```python
from build123d import *

# Parameters (mm, degrees)
SKETCH1_R           = 2.1
SKETCH1_R_2         = 12.5
SKETCH1_R_3         = 2
SKETCH1_R_4         = 2.5
SKETCH1_R_5         = 2.100093489
SKETCH1_R_6         = 2.100208614
SKETCH1_W           = 33
SKETCH1_H           = 80
BOSS_EXTRUDE1_DEPTH = 5


with BuildPart() as part:
    # Sketch1 → Boss-Extrude1 (new body)
    with BuildSketch(Plane.XY):
        with BuildLine():
            Line((101.645117601, -93.770346549), (127.497608455, -93.770346549))
            ThreePointArc((127.497608455, -93.770346549), (132.017726056, -96.632932955), (136.537843658, -93.770346549))
            Line((136.537843658, -93.770346549), (157.551292677, -93.770346549))
            Line((157.551292677, -93.770346549), (157.551292677, 97.083097938))
            Line((157.551292677, 97.083097938), (81.43113923, 97.083097938))
            ThreePointArc((81.43113923, 97.083097938), (77.101012211, 99.583097938), (72.770885192, 97.083097938))
            Line((72.770885192, 97.083097938), (36.650918722, 97.083097938))
            Line((36.650918722, 97.083097938), (-36.650918722, 97.083097938))
            Line((-36.650918722, 97.083097938), (-72.770791704, 97.083097938))
            ThreePointArc((-72.770791704, 97.083097938), (-77.100918722, 99.583097938), (-81.431045741, 97.083097938))
            Line((-81.431045741, 97.083097938), (-157.551292677, 97.083097938))
            Line((-157.551292677, 97.083097938), (-157.551292677, -93.770346549))
            Line((-157.551292677, -93.770346549), (-136.247071986, -93.770346549))
            ThreePointArc((-136.247071986, -93.770346549), (-132.0168916, -96.104718311), (-127.786711214, -93.770346549))
            Line((-127.786711214, -93.770346549), (-101.356014842, -93.770346549))
            ThreePointArc((-101.356014842, -93.770346549), (-97.125834456, -96.104718311), (-92.89565407, -93.770346549))
            Line((-92.89565407, -93.770346549), (-71.59143338, -93.770346549))
            Line((-71.59143338, -93.770346549), (-54.846081626, -64.766546521))
            ThreePointArc((-54.846081626, -64.766546521), (-52.366007385, -62.970931929), (-52.050996654, -59.925317338))
            Line((-52.050996654, -59.925317338), (-36.950417228, -33.770346549))
            Line((-36.950417228, -33.770346549), (36.950417228, -33.770346549))
            Line((36.950417228, -33.770346549), (52.039816857, -59.905953361))
            ThreePointArc((52.039816857, -59.905953361), (52.273889994, -63.173966334), (54.987035679, -65.010686103))
            Line((54.987035679, -65.010686103), (71.59143338, -93.770346549))
            Line((71.59143338, -93.770346549), (92.604882399, -93.770346549))
            ThreePointArc((92.604882399, -93.770346549), (97.125, -96.632932955), (101.645117601, -93.770346549))
        make_face()
        with Locations((20.5, 73.517875823)):
            Circle(SKETCH1_R, mode=Mode.SUBTRACT)
        with Locations((-20.5, 73.517875823)):
            Circle(SKETCH1_R, mode=Mode.SUBTRACT)
        with Locations((0, 73.517875823)):
            Circle(SKETCH1_R_2, mode=Mode.SUBTRACT)
        with Locations((36, 31.229653451)):
            Circle(SKETCH1_R_3, mode=Mode.SUBTRACT)
        with Locations((-5, -3.770346549)):
            Circle(SKETCH1_R_3, mode=Mode.SUBTRACT)
        with Locations((5, -3.770346549)):
            Circle(SKETCH1_R_3, mode=Mode.SUBTRACT)
        with Locations((36, -3.770346549)):
            Circle(SKETCH1_R_3, mode=Mode.SUBTRACT)
        with Locations((-36, 31.229653451)):
            Circle(SKETCH1_R_3, mode=Mode.SUBTRACT)
        with Locations((-5, 31.229653451)):
            Circle(SKETCH1_R_3, mode=Mode.SUBTRACT)
        with Locations((5, 31.229653451)):
            Circle(SKETCH1_R_3, mode=Mode.SUBTRACT)
        with Locations((-36, -3.770346549)):
            Circle(SKETCH1_R_3, mode=Mode.SUBTRACT)
        with Locations((93.2, 39.229653451)):
            Circle(SKETCH1_R_4, mode=Mode.SUBTRACT)
        with Locations((-93.2, 39.229653451)):
            Circle(SKETCH1_R_4, mode=Mode.SUBTRACT)
        with Locations((-93.2, -11.770346549)):
            Circle(SKETCH1_R_4, mode=Mode.SUBTRACT)
        with Locations((93.2, -11.770346549)):
            Circle(SKETCH1_R_4, mode=Mode.SUBTRACT)
        with Locations((-77.100918722, 94.583097938)):
            Circle(SKETCH1_R, mode=Mode.SUBTRACT)
        with Locations((-97.125834456, -91.104718311)):
            Circle(SKETCH1_R, mode=Mode.SUBTRACT)
        with Locations((-55.613602649, -61.095931929)):
            Circle(SKETCH1_R, mode=Mode.SUBTRACT)
        with Locations((77.101012211, 94.583097938)):
            Circle(SKETCH1_R_5, mode=Mode.SUBTRACT)
        with Locations((97.125, -91.632932955)):
            Circle(SKETCH1_R, mode=Mode.SUBTRACT)
        with Locations((55.521485258, -61.298966334)):
            Circle(SKETCH1_R, mode=Mode.SUBTRACT)
        with Locations((-0.000208614, -31.270346549)):
            Circle(SKETCH1_R_6, mode=Mode.SUBTRACT)
        with Locations((-100.592116007, -39.629860895)):
            Circle(SKETCH1_R, mode=Mode.SUBTRACT)
        with Locations((-121.092116007, -75.13690245)):
            Circle(SKETCH1_R, mode=Mode.SUBTRACT)
        with Locations((-110.842116007, -57.383381672)):
            Circle(SKETCH1_R_2, mode=Mode.SUBTRACT)
        with Locations((-132.0168916, -91.104718311)):
            Circle(SKETCH1_R, mode=Mode.SUBTRACT)
        with Locations((132.017726056, -91.632932955)):
            Circle(SKETCH1_R, mode=Mode.SUBTRACT)
        with Locations((121.092116007, -75.13690245)):
            Circle(SKETCH1_R, mode=Mode.SUBTRACT)
        with Locations((100.592116007, -39.629860895)):
            Circle(SKETCH1_R, mode=Mode.SUBTRACT)
        with Locations((110.842116007, -57.383381672)):
            Circle(SKETCH1_R_2, mode=Mode.SUBTRACT)
        with Locations((-56.5, 13.729653451)):
            Rectangle(SKETCH1_W, SKETCH1_H, mode=Mode.SUBTRACT)
        with Locations((56.5, 13.729653451)):
            Rectangle(SKETCH1_W, SKETCH1_H, mode=Mode.SUBTRACT)
        with BuildLine():
            Line((-112.97, 60.222473641), (-115.57, 60.222473641))
            ThreePointArc((-115.57, 60.222473641), (-119.105533906, 58.758007547), (-120.57, 55.222473641))
            Line((-120.57, 55.222473641), (-120.57, -27.763166739))
            ThreePointArc((-120.57, -27.763166739), (-119.105533906, -31.298700645), (-115.57, -32.763166739))
            Line((-115.57, -32.763166739), (-112.97, -32.763166739))
            ThreePointArc((-112.97, -32.763166739), (-109.434466094, -31.298700645), (-107.97, -27.763166739))
            Line((-107.97, -27.763166739), (-107.97, 55.222473641))
            ThreePointArc((-107.97, 55.222473641), (-109.434466094, 58.758007547), (-112.97, 60.222473641))
        make_face(mode=Mode.SUBTRACT)
        with BuildLine():
            Line((112.97, -32.763166739), (115.57, -32.763166739))
            ThreePointArc((115.57, -32.763166739), (119.105533906, -31.298700645), (120.57, -27.763166739))
            Line((120.57, -27.763166739), (120.57, 55.222473641))
            ThreePointArc((120.57, 55.222473641), (119.105533906, 58.758007547), (115.57, 60.222473641))
            Line((115.57, 60.222473641), (112.97, 60.222473641))
            ThreePointArc((112.97, 60.222473641), (109.434466094, 58.758007547), (107.97, 55.222473641))
            Line((107.97, 55.222473641), (107.97, -27.763166739))
            ThreePointArc((107.97, -27.763166739), (109.434466094, -31.298700645), (112.97, -32.763166739))
        make_face(mode=Mode.SUBTRACT)
    extrude(amount=BOSS_EXTRUDE1_DEPTH)


solid = part.part
```
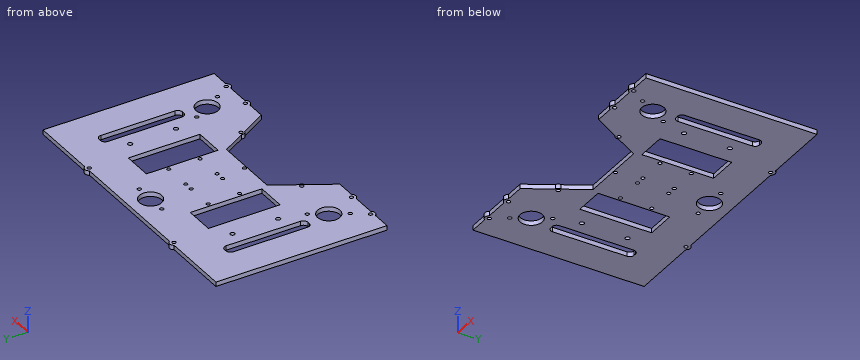
Here's how the part is built. I have some questions about the finished solid (model axes, mm). Give positions to 0.01 mm unless a question says otherwise; leave off trailing zeros. Write each loop counter-clockwise with the first axis right and the second up, starting at its lowest first coordinate (ties: lowest second). Pieces come first, ordered by that corner, then holes. Notation, with made-up numbers: (4, -12) -> (56, -12) arc R24 cw to (56, 12) -> close; hole circle Ø5 at (10, 47.25). An arc over 180 degrees is marked (long way). Write each question's results on one line, items separated by ' | '.
Item 1: Suppose I cut it at B-B on z = 0.9. Give the number of separate pieces and of enclosed holes in the cut face, plus the area to 3 significant figures.
Output:
separate pieces: 1 | enclosed holes: 34 | area: 44,300 mm^2
Item 2: If I drill on L1, parallel to X at y = 34.5, z = 3.7; L2, parallel to Y at x = 36, z = 0.35; L3, parallel to Y at x = -5, z = 2.25, over which ranges is the centre line in solid material (lowest first)?
Output:
L1: x = -157.55 to -120.57, -107.97 to -73, -40 to 40, 73 to 107.97, 120.57 to 157.55 | L2: y = -33.77 to -5.77, -1.77 to 29.23, 33.23 to 97.08 | L3: y = -33.77 to -5.77, -1.77 to 29.23, 33.23 to 62.06, 84.97 to 97.08
Item 3: For pin 1 Ø5 at (x, y) = (-100.59, -39.63) entering from +Z; pin 2 Ø3.5 at (x, y) = (-5, 31.23) entering from -Z; pin 3 Ø1.3 at (x, z) = (114, 2) entering from +Y; pin 4 Ø1.5 at (x, z) = (88.5, 3.5) entering from -Y, each with a flat end and sliding along its axis, tell me the tip position at first contact or that it passes through.
Output:
pin 1: stops at z = 5 | pin 2: passes through | pin 3: stops at y = 97.08 | pin 4: stops at y = -93.77
Item 4: Suppose I cut it at A-A on y = 50. Write out the boundary of the cut face in (x, z).
Output:
outline: (-157.55, 0) -> (-120.57, 0) -> (-120.57, 5) -> (-157.55, 5) -> close; (-107.97, 0) -> (-73, 0) -> (-73, 5) -> (-107.97, 5) -> close; (-40, 0) -> (40, 0) -> (40, 5) -> (-40, 5) -> close; (73, 0) -> (107.97, 0) -> (107.97, 5) -> (73, 5) -> close; (120.57, 0) -> (157.55, 0) -> (157.55, 5) -> (120.57, 5) -> close
